Read the model definition and answer for the solid it produces. Units are mm, in the model's axes. A direction names the side the tool comes from. Round coordinates to 2 decimals unless told otherwise and drop trailing zeros. Order: outer loops, then holes, each group sorted by start corner. A loop starts at its lowest first (then second) coordinate and runs counter-clockwise, first axis right, second up. Notation, with made-up numbers: (9.5, 10.25) - (49.5, 10.25) arc R20 ccw to (49.5, 33.25) - close; hole circle Ø3 at (-39.5, 74.5). An arc over 180 degrees is marked (long way). Answer as a JSON object with one key per item and string values. Group by question number.
Q1. A tool of negligible diameter and unlimited length cuts with its end or side. For faces 1 (the flat face through (-20.32, 7, 30)), 2 (the cylindrical face through (69.3, 52, 28.8)), from which of +Z, -Z, +X, -X, +Y, -Y can it reach the whole face along a straight path? Write none if from no direction.
Q2. Consider line 1 (X direction, y = 20, z = 17); line 2 (Y direction, x = 49.5, z = 49.5); line 3 (Z direction, x = 5.5, y = 49). Determine where each line is inside the solid, lowest interval first.
Q3. A cutting plane is placed at C-C on y = 10. Determine the outline of the cut face in (x, z).
Q4. A cutting plane is placed at A-A on z = 29.5. Determine the outline of the cut face in (x, y), and give its area (3 significant figures).
Q5. A cutting plane is placed at B-B on x = 43. Determine the outline of the cut face in (y, z).
Q6. Given pin 1 Ø10 at (x, y) = (22, 18.5) entering from +Z, flat-ended and moving along its own axis, determine where the tip first touches the part or whether it passes through.
Q7. The mould has two halves that part along X. Classify faces 3 (the cylindrical face through (-21.05, -38.17, 28.8)), 4 (the flat face through (25, 53.899, 29)), 5 (the flat face through (24, 8, 2.54)): pulls with the +X half, pulls with the -X half, needs draft (parallel to the pull), parting line crosses it, or undercut.
```python
from build123d import *

# Parameters (mm, degrees)
F1_DEPTH = 58.42
F2_T     = -2.54


with BuildPart() as f1:
    # F0 (on Top) → F1 (new body)
    with BuildSketch(Plane.XY):
        with BuildLine():
            Line((64.77, 53.898801), (-16.51, 53.898801))
            ThreePointArc((-16.51, 53.898801), (-21.000128, 52.038929), (-22.86, 47.548801))
            Line((-22.86, 47.548801), (-22.86, -33.731199))
            ThreePointArc((-22.86, -33.731199), (-21.000128, -38.221327), (-16.51, -40.081199))
            Line((-16.51, -40.081199), (64.77, -40.081199))
            ThreePointArc((64.77, -40.081199), (69.260128, -38.221327), (71.12, -33.731199))
            Line((71.12, -33.731199), (71.12, 47.548801))
            ThreePointArc((71.12, 47.548801), (69.260128, 52.038929), (64.77, 53.898801))
        make_face()
    extrude(amount=F1_DEPTH)

    # F2
    f2_openings = [f1.faces().sort_by_distance(p)[0] for p in [
        (24.13, 6.908801, 58.42),
    ]]
    offset(amount=F2_T, openings=f2_openings)


solid = f1.part
```
Result set:
{
 "1": {"face 1": "+Z", "face 2": "+Z, -Z, +X, +Y"},
 "2": {"line 1": "x = -22.86 to -20.32, 68.58 to 71.12", "line 2": "y = -40.08 to -37.54, 51.36 to 53.9", "line 3": "z = 0 to 2.54"},
 "3": {"outline": "(-22.86, 0) - (71.12, 0) - (71.12, 58.42) - (68.58, 58.42) - (68.58, 2.54) - (-20.32, 2.54) - (-20.32, 58.42) - (-22.86, 58.42) - close"},
 "4": {"outline": "(-22.86, -33.73) arc R6.35 ccw to (-16.51, -40.08) - (64.77, -40.08) arc R6.35 ccw to (71.12, -33.73) - (71.12, 47.55) arc R6.35 ccw to (64.77, 53.9) - (-16.51, 53.9) arc R6.35 ccw to (-22.86, 47.55) - close; hole (-20.32, -33.73) arc R3.81 ccw to (-16.51, -37.54) - (64.77, -37.54) arc R3.81 ccw to (68.58, -33.73) - (68.58, 47.55) arc R3.81 ccw to (64.77, 51.36) - (-16.51, 51.36) arc R3.81 ccw to (-20.32, 47.55) - close", "area": "907 mm²"},
 "5": {"outline": "(-40.08, 0) - (53.9, 0) - (53.9, 58.42) - (51.36, 58.42) - (51.36, 2.54) - (-37.54, 2.54) - (-37.54, 58.42) - (-40.08, 58.42) - close"},
 "6": {"pin 1": "stops at z = 2.54"},
 "7": {"face 3": "pulls with the -X half", "face 4": "needs draft", "face 5": "undercut"}
}
